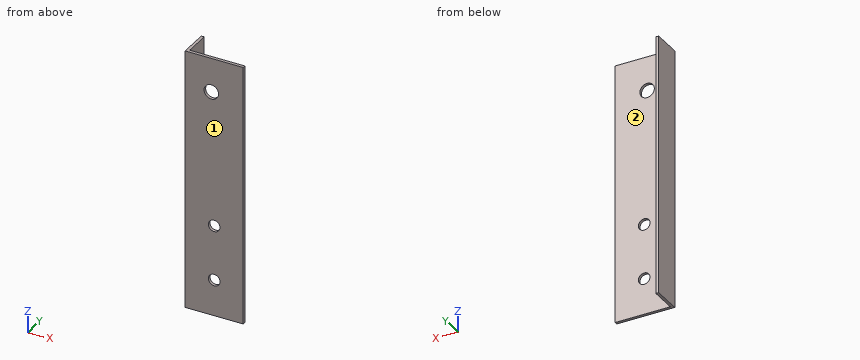
```python
from build123d import *

# Parameters (mm, degrees)
BOSS_EXTRUDE1_DEPTH = 180
SKETCH3_R           = 4
SKETCH3_R_2         = 5
CUT_EXTRUDE1_DEPTH  = 10


with BuildPart() as part:
    # Sketch1 → Boss-Extrude1 (new body)
    with BuildSketch(Plane.XY):
        Polygon((-69.579831933, 29.327731092), (-67.579831933, 29.327731092), (-67.579831933, 11.327731092), (-29.579831933, 11.327731092), (-29.579831933, 9.327731092), (-69.579831933, 9.327731092), (-69.579831933, 11.327731092), align=None)
    extrude(amount=BOSS_EXTRUDE1_DEPTH)

    # Sketch3 → Cut-Extrude1 (cut)
    with BuildSketch(Plane.XZ.offset(-9.327731092)):
        with Locations(Location((-49.579831933, 63, 0), (0, 0, 270))):
            Circle(SKETCH3_R)
        with Locations(Location((-49.579831933, 25, 0), (0, 0, 270))):
            Circle(SKETCH3_R)
        with Locations(Location((-51.579831933, 156.42594511, 0), (0, 0, 270))):
            Circle(SKETCH3_R_2)
    extrude(amount=-CUT_EXTRUDE1_DEPTH, mode=Mode.SUBTRACT)


solid = part.part
```
Source: CAD feature listing. Evaluate the final solid. Frame: model axes, mm. Face numbers are marked on the shaded views. A direction names the side the tool comes from. Give positions to 0.01 mm unless a question says otherwise; leave off trailing zeros. Loops run counter-clockwise (first coordinate to the right, second up) from the corner with the lowest first, then second, coordinate; pieces in that order, holes last. Notation, with made-up numbers: (59, -5) - (105, -5) arc R14 cw to (105, 10) - close; hole circle Ø1 at (51, 25.5). An arc over 180 degrees is marked (long way). Use CSV: the item, a comma, the result in double quotes. Start each with the question number.
1. Section C-C (y = 22). Output: boundary loops of the cut face in (x, z), then the cut area to 3 significant figures.
2. Section D-D (x = -40.5). Output: boundary loops of the cut face in (y, z), then the cut area to 3 significant figures.
3. Pin query (flat end, axial travel): pin 1 (10.5 mm diameter, centred on x = -49.58, z = 63, fed in from +Y); pin 2 (8 mm diameter, centred on y = 22, z = 107, fed in from +X); pin 3 (7 mm diameter, centred on x = -49.58, z = 25, fed in from +Y). Return the tip coordinate at first contact, or that it passes through.
4. Section A-A (z = 25). Output: boundary loops of the cut face in (x, y).
5. Ray query, L1, parallel to X at y = 10, z = 25; L2, parallel to Y at x = -50, z = 85; L3, parallel to X at y = 25.5, z = 42. Return the intervals inside material, ascending.
6. Section B-B (z = 141.5). Output: boundary loops of the cut face in (x, y).
7. Reachability of the marked faces 1 and 2 from +Z, -Z, +X, -X, +Y, -Y: full face, straight path, thin tool, end or side. Return the list, or none.
Response:
1,outline,"(-69.58, 0) - (-67.58, 0) - (-67.58, 180) - (-69.58, 180) - close"
1,area,"360 mm²"
2,outline,"(9.33, 0) - (11.33, 0) - (11.33, 180) - (9.33, 180) - close"
2,area,"360 mm²"
3,pin 1,"y = 11.33"
3,pin 2,"x = -67.58"
3,pin 3,"through"
4,outline,"(-69.58, 9.33) - (-53.58, 9.33) - (-53.58, 11.33) - (-67.58, 11.33) - (-67.58, 29.33) - (-69.58, 29.33) - close; (-45.58, 9.33) - (-29.58, 9.33) - (-29.58, 11.33) - (-45.58, 11.33) - close"
5,L1,"-69.58 to -53.58, -45.58 to -29.58"
5,L2,"9.33 to 11.33"
5,L3,"-69.58 to -67.58"
6,outline,"(-69.58, 9.33) - (-29.58, 9.33) - (-29.58, 11.33) - (-67.58, 11.33) - (-67.58, 29.33) - (-69.58, 29.33) - close"
7,face 1,"+Z, -Z, +X, -X, -Y"
7,face 2,"+Z, -Z, +X, +Y"
